The model under review builds one solid part; all positions refer to its coordinate system, in mm. Face numbers are marked on the shaded views. A direction names the side the tool comes from. Coordinates: 2 decimals unless noted, no trailing zeros. Order: outer loops, then holes, each group sorted by start corner. A loop starts at its lowest first (then second) coordinate and runs counter-clockwise, first axis right, second up. Notation, with made-up numbers: (28, -32) -> (70, -32) arc R18 ccw to (70, 1) -> close; hole circle Ø7 at (64.5, -27.75). An arc over 180 degrees is marked (long way). Use CSV: the item, a comma, the result in double quotes. Start each with the question number.
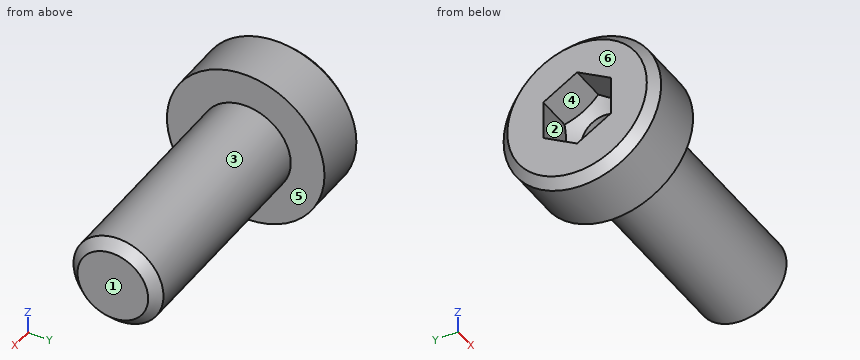
Autodesk Inventor part; units mm, degrees
ref_plane "Work Plane1" through (5, 0, 0) normal (0, 0.5, 0.866) x (1, 0, 0)
ref_plane "YZ Plane" through (0, 0, 0) normal (1, 0, 0) x (0, 1, 0)
ref_plane "XZ Plane" through (0, 0, 0) normal (0, 1, 0) x (-1, 0, 0)
sketch "Szkic1" plane through (0, 0, 0) normal (0, 0, 1) x (1, 0, 0)
  line L0 (1.0774, 0) -> (10, 0)
  line L1 (10, 0) -> (10, 2)
  line L2 (10, 2) -> (0, 2)
  line L3 (0, 2) -> (0, 3.5)
  line L4 (0, 3.5) -> (-2.8, 3.5)
  line L5 (-2.8, 3.5) -> (-2.8, 1.7321)
  line L6 (-2.8, 1.7321) -> (-1.2, 1.7321)
  line L7 (-1.2, 1.7321) -> (-0.7774, 1)
  line L8 (-5.36, 0) -> (12.56, 0)
  line L9 (0, -0.7) -> (0, 4.2)
  line L10 (-0.7774, 1) -> (0.5, 1)
  line L11 (0.5, 1) -> (1.0774, 0)
  line L12 (-2.8, 1.7321) -> (-2.8, 0) construction
  line L13 (-2.8, 3.1) -> (-2.4, 3.5)
  dimension "d0" = 2.8
  dimension "d1" = 1.6
  dimension "d2" = 60
  dimension "d3" = 4
  dimension "d4" = 3.4641
  dimension "d5" = 7
  dimension "d15" = 3.3
  dimension "d16" = 2
  dimension "d17" = 10
  dimension "d32" = 45
  dimension "d33" = 0.4
revolve "Bryła" add sketch "Szkic1" angle 360 about axis through (1.0774, 0, 0) along (1, 0, 0) contours L11 L10 L9 L2 L1 L0 | L10 L7 L6 L5 L13 L4 L3 L9 | L13 L5 L4
revolve "Faza2" cut sketch "Szkic1" angle 360 about axis through (-10, 0, 0) along (1, 0, 0) contours L13 L5 L4
sketch "Szkic2" plane through (-2.8, 0, 0) normal (-1, 0, 0) x (0, 0, 1)
  circle A0 centre (0, 0) radius 1.7321
  line L0 (0, -4.9) -> (0, 4.9)
  line L1 (-4.9, 0) -> (4.9, 0)
  line L2 (1.7321, 0) -> (0.866, -1.5)
  line L3 (0.866, -1.5) -> (-0.866, -1.5)
  line L4 (-0.866, -1.5) -> (-1.7321, 0)
  line L5 (-1.7321, 0) -> (-0.866, 1.5)
  line L6 (-0.866, 1.5) -> (0.866, 1.5)
  line L7 (0.866, 1.5) -> (1.7321, 0)
extrude "Szczelina" add sketch "Szkic2" against normal up to next contours L7 A0 | A0 L2 | L6 L0 A0 | A0 L0 L3 | L0 L6 A0 | A0 L3 L0 | L4 A0 | A0 L5
thread "Gwint"
chamfer "Faza1" distance 0.4294 distance2 0.4294 1 edges at (10, -2, 0) measured on face at (10, 0.556, 0.0273)
ref_plane "Work Plane1" through (5, 0, 0) normal (0, 0.5, 0.866) x (1, 0, 0)
equation "\"d0\" = KOH"
equation "\"d1\" = INTI"
equation "\"d3\" = GD"
equation "\"d4\" = 1.1547 * SW"
equation "\"d5\" = KOD"
equation "\"d15\" = INFT"
equation "\"d16\" = SDT"
equation "\"d17\" = NLG"
equation "\"d33\" = Cham"
equation "\"d7\" = GEL"
equation "\"d9\" = -0.5 * SPD + 0.5 * GD"
equation "\"d12\" = GUL"
equation "\"GD\" = NND"
equation "\"NLG\" = 10"
equation "\"GEL\" = 6.5"
equation "\"KOD\" = 7"
equation "\"KOH\" = 2.8"
equation "\"GUL\" = 0.61345 * PTC"
equation "\"SW\" = 3"
equation "\"INTI\" = 1.6"
equation "\"SPD\" = NND - 1.2269 * PTC"
equation "\"SDT\" = 2"
equation "\"INFT\" = 3.3"
equation "\"Cham\" = 0.4"
equation "\"TOA\" = 30deg"
equation "\"GD1\" = THREADDIA - 1.2269 * PTC"
equation "\"THREADDIA\" = 4"
equation "\"BDM\" = NND"
equation "\"FAWI\" = 45deg"
equation "\"RR\" = 0.1 * NND"
equation "\"PTC\" = 0.7"
equation "\"NND\" = 4"
equation "\"FAWI1\" = 45deg"
equation "\"GAL\" = 0.61345 * PTC"
equation "\"E0\" = 1.155 * SW"
properties part number "DIN 6912 - M4 x 10" material "Stal, miękka"
Q1. Clearance check with flat-ended pins moving along their axes: pin 1 Ø2 at (x, y) = (-1.5, -1) entering from -Z; pin 2 Ø3 at (x, y) = (0, -2) entering from +Z; pin 3 Ø1.5 at (y, z) = (2, -2.5) entering from +X. State where each tip first meets the part, or that it passes through.
Q2. Add section A-A, the plane x = 1.75. State the section outline as (y, z) points, then the cut area to 3 significant figures.
Q3. To check wall thickness, follow probe 1 along Z at (x, y) = (-0.1, 0); probe 2 along X at (y, z) = (-0.25, -3); probe 3 along Z at (x, y) = (2.5, -1). State the ranges of each line that lie inside material, in increasing order.
Q4. For the marked faces 4, 5 and 6, list the 3-axis set-ups (+Z, -Z, +X, -X, +Y, -Y) from which the entire face can be reached by the end or side of a thin tool; tool diameter is ignored.
Q5. Draft analysis for pull direction Z (two halves, no side actions). For the marked faces 1, 2 and 3, state which applies: +Z half, -Z half, draft (parallel to the pull), parting line (faces both ways), or undercut.
Answer block:
1,pin 1,"stops at z = -3.5"
1,pin 2,"stops at z = 3.46"
1,pin 3,"stops at x = 0"
2,outline,"circle Ø4 at (0, 0)"
2,area,"12.6 mm²"
3,probe 1,"z = -3.5 to -1, 1 to 3.5"
3,probe 2,"x = -2.8 to 0"
3,probe 3,"z = -1.73 to 1.73"
4,face 4,"-X"
4,face 5,"+X"
4,face 6,"+Z, -Z, -X, +Y, -Y"
5,face 1,"draft"
5,face 2,"undercut"
5,face 3,"parting line"
